Check sheet for the modelled part. Datum: model origin and axes. Units: mm. Round coordinates to 2 decimals unless told otherwise and drop trailing zeros. Order: outer loops, then holes, each group sorted by start corner. A loop starts at its lowest first (then second) coordinate and runs counter-clockwise, first axis right, second up.
Q1. Cross-section at A-A on y = 82.5. Record the cut outline in (x, z), then the cut area to 3 significant figures.
Q2. Cross-section at B-B on x = -358. Record the cut outline in (y, z).
Q3. Scan lines: probe 1 along X at (y, z) = (92, 3.8); probe 2 along Y at (x, z) = (-807, 4.85). Record each from-to range of solid material in increasing order.
Q4. Depth check by flat-ended pin: P1, Ø2.5, axis at x = 369, z = 1.5, coming from the +Y side. Enter the tip coordinate at first touch or a pass-through.
from build123d import *

# Parameters (mm, degrees)
BOSS_EXTRUDE1_DEPTH = 5


with BuildPart() as part:
    # Sketch1 → Boss-Extrude1 (new body)
    with BuildSketch(Plane.XY):
        Polygon((885, 100), (885, 60), (900, 60), (900, 20), (885, 20), (885, -20), (900, -20), (900, -60), (885, -60), (885, -100), (900, -100), (900, -140), (885, -140), (885, -180), (900, -180), (900, -225), (830, -225), (830, -220), (790, -220), (790, -225), (740, -225), (740, -220), (700, -220), (700, -225), (650, -225), (650, -220), (610, -220), (610, -225), (560, -225), (560, -220), (520, -220), (520, -225), (470, -225), (470, -220), (430, -220), (430, -225), (380, -225), (380, -220), (340, -220), (340, -225), (290, -225), (290, -220), (250, -220), (250, -225), (200, -225), (200, -220), (160, -220), (160, -225), (110, -225), (110, -220), (70, -220), (70, -225), (20, -225), (20, -220), (-20, -220), (-20, -225), (-70, -225), (-70, -220), (-110, -220), (-110, -225), (-160, -225), (-160, -220), (-200, -220), (-200, -225), (-250, -225), (-250, -220), (-290, -220), (-290, -225), (-340, -225), (-340, -220), (-380, -220), (-380, -225), (-430, -225), (-430, -220), (-470, -220), (-470, -225), (-520, -225), (-520, -220), (-560, -220), (-560, -225), (-610, -225), (-610, -220), (-650, -220), (-650, -225), (-700, -225), (-700, -220), (-740, -220), (-740, -225), (-790, -225), (-790, -220), (-830, -220), (-830, -225), (-900, -225), (-900, -180), (-885, -180), (-885, -140), (-900, -140), (-900, -100), (-885, -100), (-885, -60), (-900, -60), (-900, -20), (-885, -20), (-885, 20), (-900, 20), (-900, 60), (-885, 60), (-885, 100), (-900, 100), (-900, 140), (-885, 140), (-885, 180), (-900, 180), (-900, 225), (-830, 225), (-830, 220), (-790, 220), (-790, 225), (-740, 225), (-740, 220), (-700, 220), (-700, 225), (-650, 225), (-650, 220), (-610, 220), (-610, 225), (-560, 225), (-560, 220), (-520, 220), (-520, 225), (-470, 225), (-470, 220), (-430, 220), (-430, 225), (-380, 225), (-380, 220), (-340, 220), (-340, 225), (-290, 225), (-290, 220), (-250, 220), (-250, 225), (-200, 225), (-200, 220), (-160, 220), (-160, 225), (-110, 225), (-110, 220), (-70, 220), (-70, 225), (-20, 225), (-20, 220), (20, 220), (20, 225), (70, 225), (70, 220), (110, 220), (110, 225), (160, 225), (160, 220), (200, 220), (200, 225), (250, 225), (250, 220), (290, 220), (290, 225), (340, 225), (340, 220), (380, 220), (380, 225), (430, 225), (430, 220), (470, 220), (470, 225), (520, 225), (520, 220), (560, 220), (560, 225), (610, 225), (610, 220), (650, 220), (650, 225), (700, 225), (700, 220), (740, 220), (740, 225), (790, 225), (790, 220), (830, 220), (830, 225), (900, 225), (900, 180), (885, 180), (885, 140), (900, 140), (900, 100), align=None)
    extrude(amount=BOSS_EXTRUDE1_DEPTH)


solid = part.part
Results found:
1. outline: (-885, 0) - (885, 0) - (885, 5) - (-885, 5) - close
1. area: 8,850 mm2
2. outline: (-220, 0) - (220, 0) - (220, 5) - (-220, 5) - close
3. probe 1: x = -885 to 885
3. probe 2: y = -220 to 220
4. P1: stops at y = 220
